from build123d import *

# Parameters (mm, degrees)
CROQUIS1_R                 = 31.5
SALIENTE_EXTRUIR1_DEPTH    = 8
CORTAR_EXTRUIR2_START      = -6.7
CROQUIS2_R                 = 31.5
CROQUIS2_R_2               = 27.5
CORTAR_EXTRUIR2_DEPTH      = 6.7
CORTAR_EXTRUIR4_DEPTH      = 46.260357931
CORTAR_EXTRUIR5_DEPTH      = 46.260357931
CORTAR_EXTRUIR6_DEPTH      = 46.04875137
CORTAR_EXTRUIR7_DEPTH      = 46.04875137
CORTAR_EXTRUIR8_START      = -6.7
CORTAR_EXTRUIR8_DEPTH      = 6.7
REDONDEO1_R                = 2
SALIENTE_EXTRUIR2_DEPTH    = 1.5
CORTAR_EXTRUIR9_DEPTH      = 46.260357931
CORTAR_EXTRUIR9_DEPTH_BACK = 7
CROQUIS9_R                 = 2
SALIENTE_EXTRUIR3_DEPTH    = 6.5
CROQUIS10_R                = 5
CROQUIS10_W                = 6.5
CROQUIS10_H                = 6.5
SALIENTE_EXTRUIR5_DEPTH    = 5.3
CROQUIS10_3_W              = 6.5
CROQUIS10_3_H              = 6.5
SALIENTE_EXTRUIR6_DEPTH    = 15
CROQUIS11_R                = 3.25
SALIENTE_EXTRUIR7_DEPTH    = 37


with BuildPart() as part:
    # Croquis1 → Saliente-Extruir1 (new body)
    with BuildSketch(Plane.XY):
        Circle(CROQUIS1_R)
    extrude(amount=SALIENTE_EXTRUIR1_DEPTH)

    # Croquis2 → Cortar-Extruir2 (cut)
    with BuildSketch(Plane.XY.offset(8).offset(CORTAR_EXTRUIR2_START)):
        Circle(CROQUIS2_R)
        Circle(CROQUIS2_R_2, mode=Mode.SUBTRACT)
    extrude(amount=CORTAR_EXTRUIR2_DEPTH, mode=Mode.SUBTRACT)

    # Croquis3 → Cortar-Extruir4 (cut, through all)
    with BuildSketch(Plane.XY.offset(8)):
        with BuildLine():
            ThreePointArc((16.237061362, 17.944298212), (-0.84115789, 24.185376851), (-17.444510686, 16.77286639))
            Line((-17.444510686, 16.77286639), (-15.648176648, 15.372144095))
            Line((-15.648176648, 15.372144095), (-6.504791201, 8.242432373))
            ThreePointArc((-6.504791201, 8.242432373), (-0.3649652, 10.493655245), (5.916429122, 8.674437529))
            Line((5.916429122, 8.674437529), (14.949587988, 16.787905994))
            Line((14.949587988, 16.787905994), (16.237061362, 17.944298212))
        make_face()
        with BuildLine():
            Line((-18.722764813, 11.429187385), (-20.51909885, 12.829909679))
            ThreePointArc((-20.51909885, 12.829909679), (-23.611186728, -5.305832762), (-13.057369721, -20.375109717))
            Line((-13.057369721, -20.375109717), (-5.665387689, -8.840440166))
            ThreePointArc((-5.665387689, -8.840440166), (-10.063055085, -2.997486008), (-9.579379365, 4.299475663))
            Line((-9.579379365, 4.299475663), (-18.722764813, 11.429187385))
        make_face()
        with BuildLine():
            ThreePointArc((24.2, 0), (23.015553679, 7.4782544), (19.578157945, 14.224476493))
            Line((19.578157945, 14.224476493), (18.290684571, 13.068084275))
            Line((18.290684571, 13.068084275), (9.257525705, 4.954615809))
            ThreePointArc((9.257525705, 4.954615809), (10.184645794, 2.554014496), (10.5, 0))
            ThreePointArc((10.5, 0), (9.282826662, -4.907048927), (5.913499206, -8.676435163))
            Line((5.913499206, -8.676435163), (14.229512126, -19.574498325))
            ThreePointArc((14.229512126, -19.574498325), (21.563791335, -10.983756337), (24.2, 0))
        make_face()
    extrude(amount=-CORTAR_EXTRUIR4_DEPTH, mode=Mode.SUBTRACT)

    # Croquis3_4 → Cortar-Extruir5 (cut, through all)
    with BuildSketch(Plane.XY.offset(8)):
        with BuildLine():
            Line((-2.435503713, -10.213634107), (-2.650493565, -24.05441506))
            ThreePointArc((-2.650493565, -24.05441506), (-0.350299921, -24.197464536), (1.953070703, -24.121059571))
            Line((1.953070703, -24.121059571), (2.138825202, -10.279855386))
            ThreePointArc((2.138825202, -10.279855386), (-0.151989635, -10.498899902), (-2.435503713, -10.213634107))
        make_face()
        with BuildLine():
            Line((-2.650493565, -24.05441506), (-2.701947276, -27.366941388))
            ThreePointArc((-2.701947276, -27.366941388), (-0.398068092, -27.497118791), (1.908613915, -27.433687192))
            Line((1.908613915, -27.433687192), (1.953070703, -24.121059571))
            ThreePointArc((1.953070703, -24.121059571), (-0.350299921, -24.197464536), (-2.650493565, -24.05441506))
        make_face()
    extrude(amount=-CORTAR_EXTRUIR5_DEPTH, mode=Mode.SUBTRACT)

    # Croquis4 → Cortar-Extruir6 (cut, through all)
    with BuildSketch(Plane.XY.offset(1.3)):
        Polygon((-2.701947276, -27.366941388), (1.908613915, -27.433687192), (1.818382526, -33.666548493), (-2.792178664, -33.599802689), align=None)
    extrude(amount=-CORTAR_EXTRUIR6_DEPTH, mode=Mode.SUBTRACT)

    # Croquis5 → Cortar-Extruir7 (cut, through all)
    with BuildSketch(Plane.XY.offset(1.3)):
        with BuildLine():
            ThreePointArc((-15.166933322, 22.939357742), (-7.728074889, 26.391795288), (0.398068092, 27.497118791))
            Line((0.398068092, 27.497118791), (0.455968906, 31.496699706))
            ThreePointArc((0.455968906, 31.496699706), (-8.852158509, 30.230601875), (-17.373032714, 26.275991595))
            Line((-17.373032714, 26.275991595), (-15.166933322, 22.939357742))
        make_face()
        with BuildLine():
            ThreePointArc((0.398068092, 27.497118791), (8.488809495, 26.157027992), (15.824611578, 22.490701821))
            Line((15.824611578, 22.490701821), (18.126373262, 25.762076631))
            ThreePointArc((18.126373262, 25.762076631), (9.723545421, 29.961686609), (0.455968906, 31.496699706))
            Line((0.455968906, 31.496699706), (0.398068092, 27.497118791))
        make_face()
        with BuildLine():
            Line((21.619759605, -22.909299305), (18.874393306, -20.000181933))
            ThreePointArc((18.874393306, -20.000181933), (11.036194878, -25.188338623), (1.908613915, -27.433687192))
            Line((1.908613915, -27.433687192), (1.850534631, -31.445596219))
            ThreePointArc((1.850534631, -31.445596219), (12.487224236, -28.919184478), (21.619759605, -22.909299305))
        make_face()
        with BuildLine():
            ThreePointArc((-2.701947276, -27.366941388), (-11.760706264, -24.858314267), (-19.445436483, -19.445436483))
            Line((-19.445436483, -19.445436483), (-22.273863607, -22.273863607))
            ThreePointArc((-22.273863607, -22.273863607), (-13.319125738, -28.545593173), (-2.76002656, -31.378850415))
            Line((-2.76002656, -31.378850415), (-2.701947276, -27.366941388))
        make_face()
    extrude(amount=-CORTAR_EXTRUIR7_DEPTH, mode=Mode.SUBTRACT)

    # Croquis6 → Cortar-Extruir8 (cut)
    with BuildSketch(Plane(origin=(0, 0, 0), x_dir=(-1, 0, 0), z_dir=(0, 0, -1)).offset(CORTAR_EXTRUIR8_START)):
        with BuildLine():
            Line((-4.293632906, -9.581999607), (-14.711263483, -23.234214571))
            ThreePointArc((-14.711263483, -23.234214571), (-0.92900238, -27.484303786), (13.108789939, -24.174565691))
            Line((13.108789939, -24.174565691), (3.871385851, -9.760244443))
            ThreePointArc((3.871385851, -9.760244443), (-0.229163587, -10.497498943), (-4.293632906, -9.581999607))
        make_face()
    extrude(amount=CORTAR_EXTRUIR8_DEPTH, mode=Mode.SUBTRACT)

    # Redondeo1
    redondeo1_edges = [part.edges().sort_by_distance(p)[0] for p in [
        (1.908613915, -27.433687192, 7.35),
        (-2.701947276, -27.366941388, 7.35),
    ]]
    fillet(redondeo1_edges, radius=REDONDEO1_R)

    # Croquis7 → Saliente-Extruir2 (add)
    with BuildSketch(Plane.XY.offset(8)):
        with BuildLine():
            Line((-15.669662975, 27.326025365), (-13.458452317, 23.981660935))
            ThreePointArc((-13.458452317, 23.981660935), (0, 27.5), (13.458452317, 23.981660935))
            Line((13.458452317, 23.981660935), (15.669662975, 27.326025365))
            ThreePointArc((15.669662975, 27.326025365), (0, 31.5), (-15.669662975, 27.326025365))
        make_face()
    extrude(amount=-SALIENTE_EXTRUIR2_DEPTH)

    # Croquis8 → Cortar-Extruir9 (cut, two sides: drawn at the far end of the back side and taken through both)
    with BuildSketch(Plane.XY.offset(8).offset(-CORTAR_EXTRUIR9_DEPTH_BACK)):
        with BuildLine():
            Line((0.5, 9.994890885), (0.5, 1.936491673))
            ThreePointArc((0.5, 1.936491673), (0.861766275, 1.804815472), (1.19160121, 1.606264784))
            Line((1.19160121, 1.606264784), (6.865923152, 7.280586726))
            ThreePointArc((6.865923152, 7.280586726), (3.925056399, 9.205529646), (0.5, 9.994890885))
        make_face()
        with BuildLine():
            ThreePointArc((-1.260412408, 1.552855615), (-0.668688556, 1.884902017), (0, 2))
            Line((0, 2), (0, 10.00738946))
            ThreePointArc((0, 10.00738946), (-3.733928755, 9.284698157), (-6.928560453, 7.22100366))
            Line((-6.928560453, 7.22100366), (-1.260412408, 1.552855615))
        make_face()
        with BuildLine():
            Line((7.22100366, 6.928560453), (1.552855615, 1.260412408))
            ThreePointArc((1.552855615, 1.260412408), (1.884902017, 0.668688556), (2, 0))
            Line((2, 0), (10.00738946, 0))
            ThreePointArc((10.00738946, 0), (9.284698157, 3.733928755), (7.22100366, 6.928560453))
        make_face()
        with BuildLine():
            Line((9.994890885, -0.5), (1.936491673, -0.5))
            ThreePointArc((1.936491673, -0.5), (1.804815472, -0.861766275), (1.606264784, -1.19160121))
            Line((1.606264784, -1.19160121), (7.280586726, -6.865923152))
            ThreePointArc((7.280586726, -6.865923152), (9.205529646, -3.925056399), (9.994890885, -0.5))
        make_face()
        with BuildLine():
            Line((6.928560453, -7.22100366), (1.260412408, -1.552855615))
            ThreePointArc((1.260412408, -1.552855615), (0.668688556, -1.884902017), (0, -2))
            Line((0, -2), (0, -10.00738946))
            ThreePointArc((0, -10.00738946), (3.733928755, -9.284698157), (6.928560453, -7.22100366))
        make_face()
        with BuildLine():
            ThreePointArc((-0.5, -1.936491673), (-0.861766275, -1.804815472), (-1.19160121, -1.606264784))
            Line((-1.19160121, -1.606264784), (-6.865923152, -7.280586726))
            ThreePointArc((-6.865923152, -7.280586726), (-3.925056399, -9.205529646), (-0.5, -9.994890885))
            Line((-0.5, -9.994890885), (-0.5, -1.936491673))
        make_face()
        with BuildLine():
            ThreePointArc((-1.552855615, -1.260412408), (-1.884902017, -0.668688556), (-2, 0))
            Line((-2, 0), (-10.00738946, 0))
            ThreePointArc((-10.00738946, 0), (-9.284698157, -3.733928755), (-7.22100366, -6.928560453))
            Line((-7.22100366, -6.928560453), (-1.552855615, -1.260412408))
        make_face()
        with BuildLine():
            ThreePointArc((-1.936491673, 0.5), (-1.804815472, 0.861766275), (-1.606264784, 1.19160121))
            Line((-1.606264784, 1.19160121), (-7.280586726, 6.865923152))
            ThreePointArc((-7.280586726, 6.865923152), (-9.205529646, 3.925056399), (-9.994890885, 0.5))
            Line((-9.994890885, 0.5), (-1.936491673, 0.5))
        make_face()
    extrude(amount=CORTAR_EXTRUIR9_DEPTH + CORTAR_EXTRUIR9_DEPTH_BACK, mode=Mode.SUBTRACT)

    # Croquis9 → Saliente-Extruir3 (add)
    with BuildSketch(Plane.XY.offset(8)):
        Circle(CROQUIS9_R)
    extrude(amount=SALIENTE_EXTRUIR3_DEPTH)

    # Croquis10 → Saliente-Extruir5 (add)
    with BuildSketch(Plane(origin=(0, 0, 0), x_dir=(-1, 0, 0), z_dir=(0, 0, -1))):
        Circle(CROQUIS10_R)
        Rectangle(CROQUIS10_W, CROQUIS10_H, mode=Mode.SUBTRACT)
    extrude(amount=SALIENTE_EXTRUIR5_DEPTH)

    # Croquis10_3 → Saliente-Extruir6 (add)
    with BuildSketch(Plane(origin=(0, 0, 0), x_dir=(-1, 0, 0), z_dir=(0, 0, -1))):
        Rectangle(CROQUIS10_3_W, CROQUIS10_3_H)
    extrude(amount=SALIENTE_EXTRUIR6_DEPTH)

    # Croquis11 → Saliente-Extruir7 (add)
    with BuildSketch(Plane(origin=(0, 0, -15), x_dir=(-1, 0, 0), z_dir=(0, 0, -1))):
        Circle(CROQUIS11_R)
    extrude(amount=SALIENTE_EXTRUIR7_DEPTH)


solid = part.part
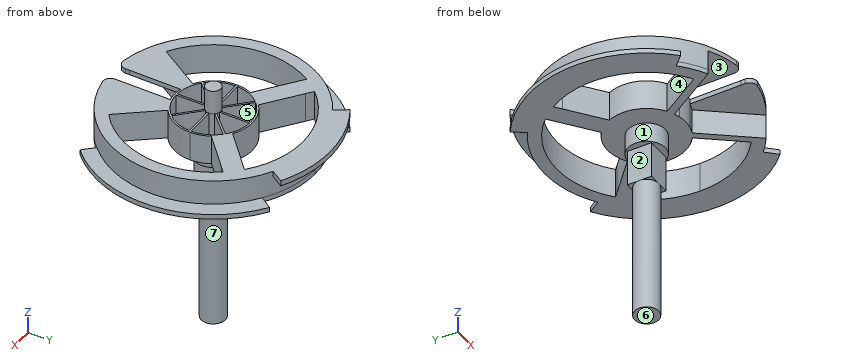
Geometry check sheet. Reference: the model listing, model coordinates, mm. Face numbers are marked on the shaded views. A direction names the side the tool comes from. Coordinates: 2 decimals unless noted, no trailing zeros. Loops run counter-clockwise (first coordinate to the right, second up) from the corner with the lowest first, then second, coordinate; pieces in that order, holes last. Notation, with made-up numbers: (56, 1) - (107, 1) arc R21 cw to (107, 33) - close; hole circle Ø2 at (-34.75, 88). An arc over 180 degrees is marked (long way). Use one line per item in the form item = value. Start each with the question number.
Item 1: Mould release check, pull along Y, two halves, no side actions. Record for the marked faces 5, 6 and 7: +Y half, -Y half, draft (parallel to the pull), parting line (faces both ways), or undercut.
Item 2: Section check B-B, the plane y = -14.5. Enter the section's corners in (x, z).
Item 3: Thickness scan on probe 1 along X at (y, z) = (11, 2); probe 2 along Y at (x, z) = (-11.5, 1); probe 3 along Z at (x, y) = (1.5, 2). Record the ranges inside material, lowest first.
Item 4: Section check C-C, the plane z = -44. Enter the section's corners in (x, y), and give its area (3 significant figures).
Item 5: Gauge pin test, flat ends, axial feed: pin 1 (3.5 mm diameter, centred on x = -7.5, y = -4, fed in from +Z); pin 2 (2 mm diameter, centred on x = -5.5, z = 5, fed in from +Y); pin 3 (7.5 mm diameter, centred on y = 4.5, z = 6, fed in from -X); pin 4 (8 mm diameter, centred on x = -12, z = -7, fed in from -Y). Record the tip position at first contact, or that the pin passes through.
Item 6: Section check A-A, the plane y = 21. Enter the section's corners in (x, z), and give its area (3 significant figures).
Item 7: Tool access check on the marked faces 1, 2, 3 and 4. Record the directions out of +Z, -Z, +X, -X, +Y, -Y that give a thin tool (end or side, any length) a straight path to the whole face; none if there is none.
Computed:
q1.face_5 = undercut
q1.face_6 = draft
q1.face_7 = parting line
q2.outline = (-27.96, 0) - (-19.37, 0) - (-19.37, 8) - (-23.37, 8) - (-23.37, 1.3) - (-27.96, 1.3) - close; (-9.29, 0) - (-6.91, 0) - (-6.91, 6.7) - (-2.5, 6.7) - (-2.5, 8) - (-9.29, 8) - close; (2.08, 6.7) - (8.05, 6.7) - (8.05, 0) - (10.36, 0) - (10.36, 8) - (2.08, 8) - close; (19.37, 0) - (27.96, 0) - (27.96, 1.3) - (23.37, 1.3) - (23.37, 8) - (19.37, 8) - close
q3.probe_1 = -25.2 to -21.56, -18.17 to -10.04, 8.51 to 15.99, 21.56 to 25.2
q3.probe_2 = -21.66 to -17.94, 5.8 to 12.14, 21.29 to 24.98
q3.probe_3 = -52 to 1
q4.outline = circle Ø6.5 at (0, 0)
q4.area = 33.2 mm2
q5.pin_1 = 8
q5.pin_2 = 27.13
q5.pin_3 = -27.49
q5.pin_4 = through
q6.outline = (-23.48, 0) - (-12.03, 0) - (-12.03, 8) - (-17.76, 8) - (-17.76, 1.3) - (-23.48, 1.3) - close; (12.03, 0) - (23.48, 0) - (23.48, 1.3) - (17.76, 1.3) - (17.76, 8) - (12.03, 8) - close
q6.area = 107 mm2
q7.face_1 = -Z
q7.face_2 = -Z, -X, +Y, -Y
q7.face_3 = -Z, -Y
q7.face_4 = +Z, -Z
